Source: three-view drawing plus pictorial views. Frame: mm from the lowest corner of the part. Round coordinates to 2 decimals unless told otherwise and drop trailing zeros. Write each loop counter-clockwise with the first axis right and the second up, starting at its lowest first coordinate (ties: lowest second). Pieces come first, ordered by that corner, then holes. Notation, with made-up numbers: (-3, 26) -> (31, 26) arc R18 cw to (31, 60) -> close; hole circle Ø7 at (7.25, 14). An arc over 180 degrees is marked (long way). Put each result on its own line as item: value.
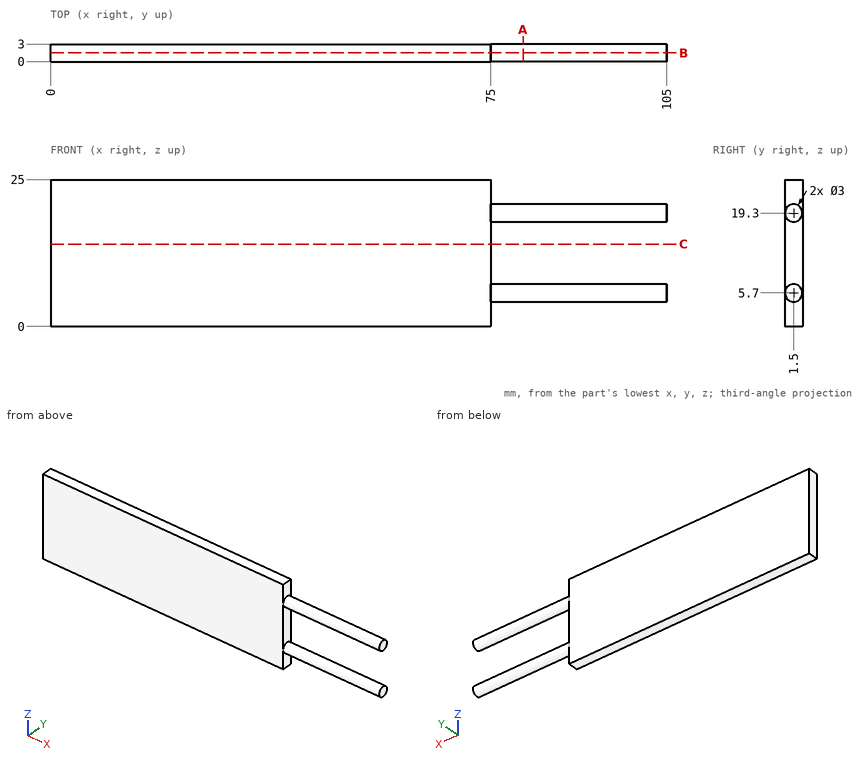
Q1. Cut plane A-A on x = 80.5. Output: boundary loops of the cut face in (y, z).
Ans:
outline: circle Ø3 at (1.5, 5.7); circle Ø3 at (1.5, 19.3)
Q2. Material intervals for line 1 (Z direction, x = 78.5, y = 1.3); line 2 (X direction, y = 2.75, z = 4.25), sorted ascending. Write a range as [from, to].
Ans:
line 1: z = [4.21, 7.19], [17.81, 20.79]
line 2: x = [0, 75]
Q3. Cut plane B-B on y = 1.5. Output: boundary loops of the cut face in (x, z), and give its area (4 significant figures).
Ans:
outline: (0, 0) -> (75, 0) -> (75, 4.2) -> (105, 4.2) -> (105, 7.2) -> (75, 7.2) -> (75, 17.8) -> (105, 17.8) -> (105, 20.8) -> (75, 20.8) -> (75, 25) -> (0, 25) -> close
area: 2,055 mm^2
Q4. Pin query (flat end, axial travel): pin 1 (1 mm diameter, centred on x = 79.5, y = 2, fed in from +Z). Return the tip coordinate at first contact, or that it passes through.
Ans:
pin 1: stops at z = 20.8
Q5. Cut plane C-C on z = 14. Output: boundary loops of the cut face in (x, y).
Ans:
outline: (0, 0) -> (75, 0) -> (75, 3) -> (0, 3) -> close
